Geometry check sheet. Reference: drawing and pictorial views, mm from the part's lowest x, y, z. Round coordinates to 2 decimals unless told otherwise and drop trailing zeros. Loops run counter-clockwise (first coordinate to the right, second up) from the corner with the lowest first, then second, coordinate; pieces in that order, holes last. Notation, with made-up numbers: (-28.5, 58) - (-9.5, 58) arc R37 ccw to (-9.5, 96) - close; hole circle Ø11 at (78.25, -17.75). An arc over 180 degrees is marked (long way). Answer as CSV lines item,"result". Start each with the question number.
1) Cross-section at D-D on y = 9. Record the boundary of the cut face in (x, z), and give its area (3 significant figures).
2) Cross-section at A-A on y = 25.2. Record the boundary of the cut face in (x, z), and give its area (3 significant figures).
3) Thickness scan on line 1 along Y through (x, z) = (4.25, 2.5); line 2 along X through (y, z) = (25.2, 3.35); line 3 along X through (y, z) = (31.5, 4.25). Record the ranges inside material, lowest first.
4) Cross-section at B-B on x = 3.5. Record the boundary of the cut face in (y, z), and give its area (3 significant figures).
5) Draft check along X on the marked faces 1, 2, 3 and 4. Enter one of: released by +X, released by -X, zero draft, split by the parting line, or undercut.
6) Cross-section at C-C on z = 4. Record the boundary of the cut face in (x, y), and give its area (3 significant figures).
7) Depth check by flat-ended pin: P1, Ø1, axis at y = 13, z = 5.5, coming from the -X side; P2, Ø2, axis at x = 3.5, y = 26, coming from the +Z side; P3, Ø1.5, axis at x = 2.5, y = 13, coming from the +Z side; P4, Ø4, axis at x = 3.9, y = 31.8, coming from the +Z side. Enter the tip coordinate at first touch or a pass-through.
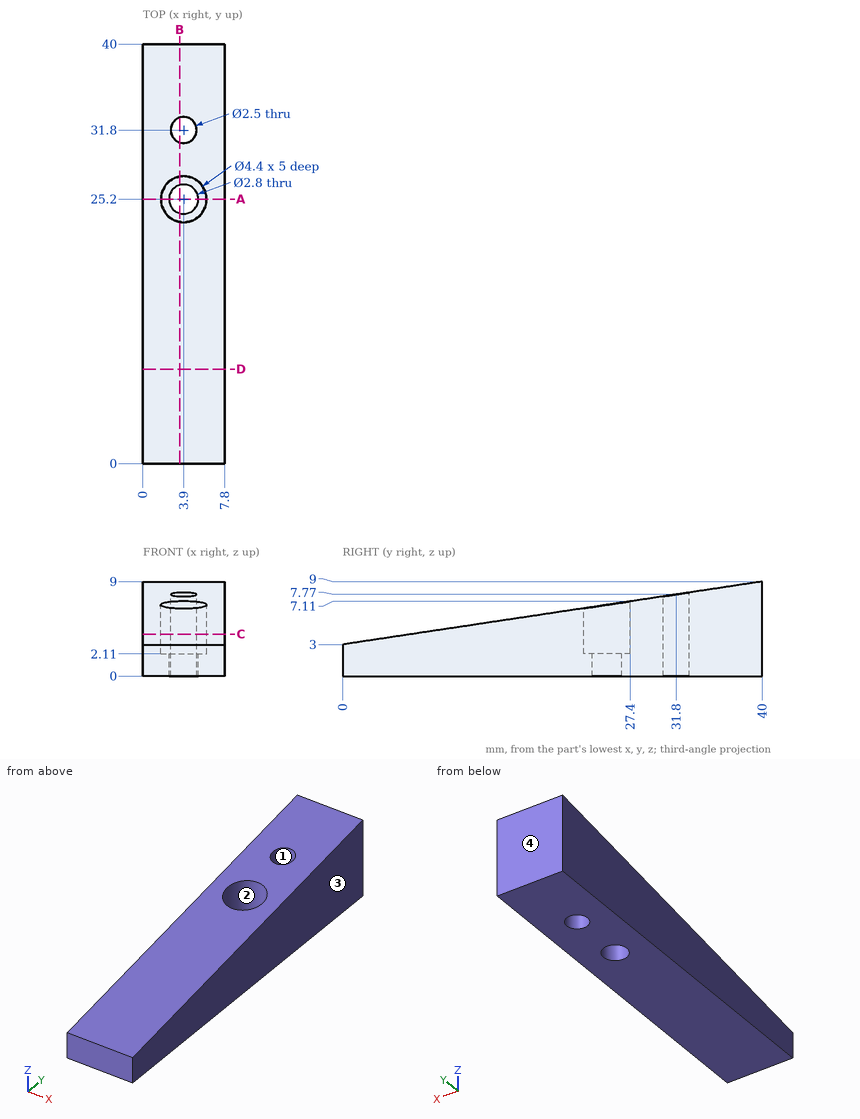
Answer block:
1,outline,"(0, 0) - (7.8, 0) - (7.8, 4.35) - (0, 4.35) - close"
1,area,"33.9 mm^2"
2,outline,"(0, 0) - (2.5, 0) - (2.5, 2.11) - (1.7, 2.11) - (1.7, 6.78) - (0, 6.78) - close; (5.3, 0) - (7.8, 0) - (7.8, 6.78) - (6.1, 6.78) - (6.1, 2.11) - (5.3, 2.11) - close"
2,area,"26.4 mm^2"
3,line 1,"y = 0 to 23.03, 27.37 to 30.6, 33 to 40"
3,line 2,"x = 0 to 1.7, 6.1 to 7.8"
3,line 3,"x = 0 to 2.69, 5.11 to 7.8"
4,outline,"(0, 0) - (23.86, 0) - (23.86, 2.11) - (23.04, 2.11) - (23.04, 6.46) - (0, 3) - close; (26.54, 0) - (30.62, 0) - (30.62, 7.59) - (27.36, 7.1) - (27.36, 2.11) - (26.54, 2.11) - close; (32.98, 0) - (40, 0) - (40, 9) - (32.98, 7.95) - close"
4,area,"196 mm^2"
5,face 1,"undercut"
5,face 2,"undercut"
5,face 3,"released by +X"
5,face 4,"zero draft"
6,outline,"(0, 6.67) - (7.8, 6.67) - (7.8, 40) - (0, 40) - close; hole circle Ø4.4 at (3.9, 25.2); hole circle Ø2.5 at (3.9, 31.8)"
6,area,"240 mm^2"
7,P1,"passes through"
7,P2,"stops at z = 2.11"
7,P3,"stops at z = 5.06"
7,P4,"stops at z = 8.07"
